Build history of the part. All positions in model axes, mm. Round coordinates to 2 decimals unless told otherwise and drop trailing zeros. Order: outer loops, then holes, each group sorted by start corner. A loop starts at its lowest first (then second) coordinate and runs counter-clockwise, first axis right, second up. Notation, with made-up numbers: M 52,-12 L 94,-12 A30 ccw 94,12 Z; hole C -18,20.5 d6. An arc over 180 degrees is marked long. One line per question, with ' | ' between items. Start each with the question number.
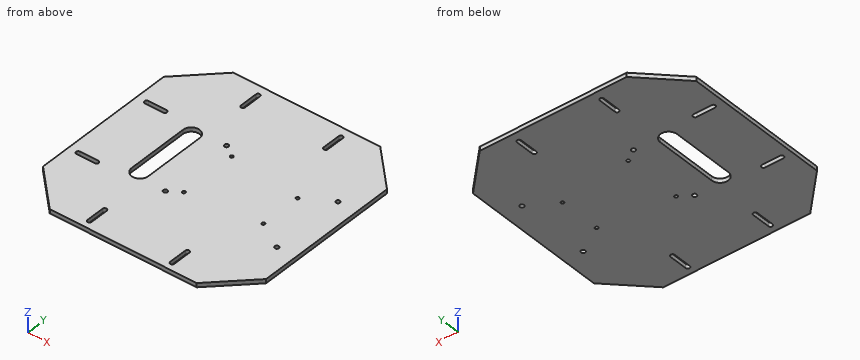
from build123d import *

# Parameters (mm, degrees)
SKETCH1_R           = 1.5
SKETCH1_R_2         = 2
BOSS_EXTRUDE2_DEPTH = 4


with BuildPart() as part:
    # Sketch1 → Boss-Extrude2 (new body)
    with BuildSketch(Plane.XY):
        Polygon((-73.597643579, 117.281365478), (67.863251178, 117.281365478), (104.632803799, 80.511812856), (104.632803799, -60.949081901), (67.894125273, -97.50252168), (-73.566769484, -97.50252168), (-110.367196201, -60.702096755), (-110.367196201, 80.511812856), align=None)
        with Locations((-9.717773474, 37.825883079)):
            Circle(SKETCH1_R, mode=Mode.SUBTRACT)
        with Locations((60.282226526, 29.825883079)):
            Circle(SKETCH1_R, mode=Mode.SUBTRACT)
        with Locations((60.282226526, -10.174116921)):
            Circle(SKETCH1_R, mode=Mode.SUBTRACT)
        with Locations((-9.717773474, -18.174116921)):
            Circle(SKETCH1_R, mode=Mode.SUBTRACT)
        with Locations((-21.13184974, 45.601933923)):
            Circle(SKETCH1_R_2, mode=Mode.SUBTRACT)
        with Locations((86.196302793, 45.601933923)):
            Circle(SKETCH1_R_2, mode=Mode.SUBTRACT)
        with Locations((86.196302793, -25.950167766)):
            Circle(SKETCH1_R_2, mode=Mode.SUBTRACT)
        with Locations((-21.13184974, -25.950167766)):
            Circle(SKETCH1_R_2, mode=Mode.SUBTRACT)
        with BuildLine():
            Line((-58.385806079, -20.095141949), (-58.385806079, 39.904858051))
            ThreePointArc((-58.385806079, 39.904858051), (-50.403357017, 47.887307113), (-42.420907955, 39.904858051))
            Line((-42.420907955, 39.904858051), (-42.420907955, -20.095141949))
            ThreePointArc((-42.420907955, -20.095141949), (-50.403357017, -28.077591011), (-58.385806079, -20.095141949))
        make_face(mode=Mode.SUBTRACT)
        with BuildLine():
            Line((-43.951300834, 90.135788358), (-43.951300834, 107.780882998))
            ThreePointArc((-43.951300834, 107.780882998), (-41.951300834, 109.780882998), (-39.951300834, 107.780882998))
            Line((-39.951300834, 107.780882998), (-39.951300834, 90.135788358))
            ThreePointArc((-39.951300834, 90.135788358), (-41.951300834, 88.135788358), (-43.951300834, 90.135788358))
        make_face(mode=Mode.SUBTRACT)
        with BuildLine():
            Line((39.83957888, 89.970561723), (39.910868679, 107.61551235))
            ThreePointArc((39.910868679, 107.61551235), (37.918965413, 109.623576437), (35.910901326, 107.63167317))
            Line((35.910901326, 107.63167317), (35.839611526, 89.986722543))
            ThreePointArc((35.839611526, 89.986722543), (37.831514793, 87.978658457), (39.83957888, 89.970561723))
        make_face(mode=Mode.SUBTRACT)
        with BuildLine():
            Line((-83.098126059, -33.179247031), (-100.743220699, -33.179247031))
            ThreePointArc((-100.743220699, -33.179247031), (-102.743220699, -31.179247031), (-100.743220699, -29.179247031))
            Line((-100.743220699, -29.179247031), (-83.098126059, -29.179247031))
            ThreePointArc((-83.098126059, -29.179247031), (-81.098126059, -31.179247031), (-83.098126059, -33.179247031))
        make_face(mode=Mode.SUBTRACT)
        with BuildLine():
            Line((-82.932899424, 50.611632682), (-100.577850051, 50.682922481))
            ThreePointArc((-100.577850051, 50.682922481), (-102.585914138, 48.691019215), (-100.594010871, 46.682955128))
            Line((-100.594010871, 46.682955128), (-82.949060244, 46.611665329))
            ThreePointArc((-82.949060244, 46.611665329), (-80.940996157, 48.603568595), (-82.932899424, 50.611632682))
        make_face(mode=Mode.SUBTRACT)
        with BuildLine():
            Line((40.21690933, -72.326072256), (40.21690933, -89.971166897))
            ThreePointArc((40.21690933, -89.971166897), (38.21690933, -91.971166897), (36.21690933, -89.971166897))
            Line((36.21690933, -89.971166897), (36.21690933, -72.326072256))
            ThreePointArc((36.21690933, -72.326072256), (38.21690933, -70.326072256), (40.21690933, -72.326072256))
        make_face(mode=Mode.SUBTRACT)
        with BuildLine():
            Line((-43.573970383, -72.160845622), (-43.645260182, -89.805796249))
            ThreePointArc((-43.645260182, -89.805796249), (-41.653356916, -91.813860335), (-39.645292829, -89.821957069))
            Line((-39.645292829, -89.821957069), (-39.574003029, -72.177006442))
            ThreePointArc((-39.574003029, -72.177006442), (-41.565906296, -70.168942355), (-43.573970383, -72.160845622))
        make_face(mode=Mode.SUBTRACT)
    extrude(amount=BOSS_EXTRUDE2_DEPTH)


solid = part.part
Item 1: Cut at D-D on x = 71.5. Write the cut outline in (y, z), then the cut area to 3 significant figures.
Item 2: Cut at B-B on y = -75. Write the cut outline in (x, z).
Item 3: Flat gauge pin, fed straight in: pin 1 (1.2 mm diameter, centred on x = -93.5, z = 1, fed in from +Y). Where does the tip first touch, or does it go through?
Item 4: Cut at A-A on y = 8.5. Write the cut outline in (x, z), then the cut area to 3 significant figures.
Item 5: Wall check: line 1 along X through (y, z) = (-88, 0.2); line 2 along X through (y, z) = (-7, 1.4); line 3 along X through (y, z) = (43, 1.9). Give the ranges that are in metal, low to high. Write a range as [from, to].
Item 6: Cut at C-C on z = 2.8. Count the separate pieces of the cut face and the enclosed holes in it, then the cut area to 3 significant figures.
Results found:
1) outline: M -93.91,0 L 113.64,0 L 113.64,4 L -93.91,4 Z | area: 830 mm^2
2) outline: M -96.07,0 L -43.59,0 L -43.59,4 L -96.07,4 Z; M -39.59,0 L 36.22,0 L 36.22,4 L -39.59,4 Z; M 40.22,0 L 90.51,0 L 90.51,4 L 40.22,4 Z
3) pin 1: stops at y = 97.98
4) outline: M -110.37,0 L -58.39,0 L -58.39,4 L -110.37,4 Z; M -42.42,0 L 104.63,0 L 104.63,4 L -42.42,4 Z | area: 796 mm^2
5) line 1: x = [-83.07, -43.64], [-39.64, 36.22], [40.22, 77.44] | line 2: x = [-110.37, -58.39], [-42.42, 104.63] | line 3: x = [-110.37, -57.76], [-43.05, 104.63]
6) separate pieces: 1 | enclosed holes: 15 | area: 41,700 mm^2
